from build123d import *

# Parameters (mm, degrees)
BOSS_EXTRUDE1_DEPTH = 10
BOSS_EXTRUDE2_DEPTH = 40


with BuildPart() as part:
    # Sketch2 → Boss-Extrude1 (new body)
    with BuildSketch(Plane(origin=(0, 0, 0), x_dir=(1, 0, 0), z_dir=(0, 1, 0))):
        Polygon((-174.250613401, -235), (-174.250613401, -250), (174.250613401, -250), (174.250613401, -235), (235, -235), (235, -174.250613401), (250, -174.250613401), (250, 174.250613401), (235, 174.250613401), (235, 235), (174.250613401, 235), (174.250613401, 250), (-174.250613401, 250), (-174.250613401, 235), (-235, 235), (-235, 174.250613401), (-250, 174.250613401), (-250, -174.250613401), (-235, -174.250613401), (-235, -235), align=None)
        Polygon((174.250613401, -235), (174.250613401, -250), (250, -250), (250, -174.250613401), (235, -174.250613401), (235, -235), align=None)
        Polygon((-250, -174.250613401), (-250, -250), (-174.250613401, -250), (-174.250613401, -235), (-235, -235), (-235, -174.250613401), align=None)
        Polygon((-250, 216.633029877), (-250, 174.250613401), (-235, 174.250613401), (-235, 235), (-174.250613401, 235), (-174.250613401, 250), (-216.633029877, 250), (-250, 250), align=None)
        Polygon((235, 174.250613401), (250, 174.250613401), (250, 250), (174.250613401, 250), (174.250613401, 235), (235, 235), align=None)
    extrude(amount=BOSS_EXTRUDE1_DEPTH)

    # Sketch2_3 → Boss-Extrude2 (add)
    with BuildSketch(Plane(origin=(0, 0, 0), x_dir=(1, 0, 0), z_dir=(0, 1, 0))):
        Polygon((-250, -174.250613401), (-250, -250), (-174.250613401, -250), (-174.250613401, -235), (-235, -235), (-235, -174.250613401), align=None)
        Polygon((174.250613401, -235), (174.250613401, -250), (250, -250), (250, -174.250613401), (235, -174.250613401), (235, -235), align=None)
        Polygon((-250, 250), (-250, 174.250613401), (-235, 174.250613401), (-235, 235), (-174.250613401, 235), (-174.250613401, 250), align=None)
        Polygon((235, 174.250613401), (250, 174.250613401), (250, 250), (174.250613401, 250), (174.250613401, 235), (235, 235), align=None)
    extrude(amount=-BOSS_EXTRUDE2_DEPTH)


solid = part.part
Work out the finished part from the listing and answer in its coordinate system (mm). A direction names the side the tool comes from. Coordinates: 2 decimals unless noted, no trailing zeros. Write each loop counter-clockwise with the first axis right and the second up, starting at its lowest first coordinate (ties: lowest second). Pieces come first, ordered by that corner, then holes. Notation, with made-up numbers: M 86.5,76.25 L 136.5,76.25 A16 ccw 136.5,89.25 Z; hole C 75,-35.5 d2. An arc over 180 degrees is marked long. Answer as CSV lines item,"result". Start each with the question number.
Item 1: Section B-B on x = -199 is taken. Write down the section's boundary in (y, z), and give its area (3 significant figures).
Item 2: Section D-D on x = 71.5 is taken. Write down the section's boundary in (y, z), and give its area (3 significant figures).
Item 3: Flat-ended cylindrical pins translate along their axes: P1, Ø5, axis at y = -3.5, z = -163, coming from the -X side; P2, Ø3, axis at x = 69.5, z = -82.5, coming from the -Y side. Find the tip coordinate at first contact, or state that the pin passes through.
Item 4: Section C-C on z = 219.5 is taken. Write down the section's boundary in (x, y), and give its area (3 significant figures).
Item 5: Section A-A on y = -23 is taken. Write down the section's boundary in (x, z), and give its area (3 significant figures).
Item 6: A tool of negligible diameter and unlimited length cuts with its end or side. For faces 1 (the face through (-204, -20, 235)), 2 (the face through (-238, -40, 228)), 3 (the face through (174.251, -20, -243)), 4 (the face through (243, -20, 174.251)), from which of +Z, -Z, +X, -X, +Y, -Y can it reach the whole face along a straight path? Write none if from no direction.
Item 7: Consider L1, parallel to Z at x = 192.5, y = -31; L2, parallel to Y at x = -72, z = 220. Determine where each line is inside the solid, lowest interval first.
Checks:
1,outline,"M -40,-250 L 10,-250 L 10,250 L -40,250 L -40,235 L 0,235 L 0,-235 L -40,-235 Z"
1,area,"6,200 mm²"
2,outline,"M 0,-250 L 10,-250 L 10,250 L 0,250 Z"
2,area,"5,000 mm²"
3,P1,"passes through"
3,P2,"stops at y = 0"
4,outline,"M -250,-40 L -235,-40 L -235,0 L 235,0 L 235,-40 L 250,-40 L 250,10 L -250,10 Z"
4,area,"6,200 mm²"
5,outline,"M -250,-250 L -174.25,-250 L -174.25,-235 L -235,-235 L -235,-174.25 L -250,-174.25 Z; M -250,174.25 L -235,174.25 L -235,235 L -174.25,235 L -174.25,250 L -250,250 Z; M 174.25,-250 L 250,-250 L 250,-174.25 L 235,-174.25 L 235,-235 L 174.25,-235 Z; M 174.25,235 L 235,235 L 235,174.25 L 250,174.25 L 250,250 L 174.25,250 Z"
5,area,"8,190 mm²"
6,face 1,"-Y"
6,face 2,"+Z, -Z, +X, -X, -Y"
6,face 3,"+Z, -Z, -Y"
6,face 4,"+X, -X, -Y"
7,L1,"z = -250 to -235, 235 to 250"
7,L2,"y = 0 to 10"
